Geometry: final body of the model. Coordinates: model frame, mm. A direction names the side the tool comes from. Round coordinates to 2 decimals unless told otherwise and drop trailing zeros. Write each loop counter-clockwise with the first axis right and the second up, starting at its lowest first coordinate (ties: lowest second). Pieces come first, ordered by that corner, then holes. Notation, with made-up numbers: (-9.5, -27) - (49.5, -27) arc R22 cw to (49.5, -14) - close; hole circle Ø1 at (49, -20). An arc over 180 degrees is marked (long way). Use a Markdown table: item, result. Add a question column.
```python
from build123d import *

# Parameters (mm, degrees)
PAD_DEPTH     = 101.6
SKETCH001_W   = 2.54
SKETCH001_H   = 83.8962
SKETCH001_W_2 = 12.7
SKETCH001_H_2 = 50.8
SKETCH001_W_3 = 146.9
SKETCH001_H_3 = 2.54
PAD001_DEPTH  = 2.54
CHAMFER_SIZE  = 50.8
FILLET_R      = 1.27


with BuildPart() as part:
    # Sketch → Pad (new body)
    with BuildSketch(Plane.XY):
        Polygon((-2.54, 2.54), (-2.54, -121.9962), (0, -121.9962), (0, 0), (185, 0), (185, -121.9962), (187.54, -121.9962), (187.54, 2.54), align=None)
    extrude(amount=PAD_DEPTH)

    # Sketch001 → Pad001 (join)
    with BuildSketch(Plane.XY):
        with Locations((1.27, -60.9981)):
            Rectangle(SKETCH001_W, SKETCH001_H)
        with Locations((178.65, -76.2)):
            Rectangle(SKETCH001_W_2, SKETCH001_H_2)
        with Locations((92.5, -1.27)):
            Rectangle(SKETCH001_W_3, SKETCH001_H_3)
    extrude(amount=PAD001_DEPTH)

    # Chamfer
    chamfer_edges = [part.edges().sort_by_distance(p)[0] for p in [
        (-1.27, -121.9962, 101.6),
        (186.27, -121.9962, 101.6),
    ]]
    chamfer(chamfer_edges, length=CHAMFER_SIZE)

    # Fillet
    fillet_edges = [part.edges().sort_by_distance(p)[0] for p in [
        (185, 0, 50.8),
        (0, 0, 50.8),
        (-2.54, 2.54, 50.8),
        (187.54, 2.54, 50.8),
    ]]
    fillet(fillet_edges, radius=FILLET_R)


solid = part.part
```
1) Pin query (flat end, axial travel): P1, Ø6, axis at x = 22, z = 36.5, coming from the -Y side; P2, Ø0.8, axis at x = 126.5, y = -1.5, coming from the +Z side; P3, Ø2, axis at x = 105, z = 1, coming from the -Y side. Return the tip coordinate at first contact, or that it passes through.
2) Section C-C, the plane z = 31.5. Return the cut outline in (x, y), then the cut area to 3 significant figures.
3) Set-up query: faces 1 (the flat face through (179, -76, 2.54)), 2 (the flat face through (186.252, -96.952, 75.844)). Return all of +Z, -Z, +X, -X, +Y, -Y with unobstructed straight access to the full face (end or side cutting, diameter ignored); none if empty.
4) Section B-B, the plane y = -62.5. Return the cut outline in (x, z).
5) Draft query along X for faces 3 (the flat face through (94, 2.54, 50)), 4 (the flat face through (187.54, -61, 50)), 5 (the flat face through (0, -62, 50)). Return one class per face: released by +X, released by -X, zero draft, split by the parting line, or undercut.
6) Section D-D, the plane x = 122.5. Return the cut outline in (y, z).
7) Section A-A, the plane y = -14.5. Return the cut outline in (x, z), then the cut area to 3 significant figures.
8) Material intervals for L1, parallel to X at y = -110.5, z = 45.5; L2, parallel to Y at x = 147, z = 46.5, sorted ascending. Write a range as from..to.
Output values:
| question | item | result |
|---|---|---|
| 1 | P1 | stops at y = 0 |
| 1 | P2 | stops at z = 2.54 |
| 1 | P3 | stops at y = -2.54 |
| 2 | outline | (-2.54, -122) - (0, -122) - (0, -1.27) arc R1.27 cw to (1.27, 0) - (183.73, 0) arc R1.27 cw to (185, -1.27) - (185, -122) - (187.54, -122) - (187.54, 1.27) arc R1.27 ccw to (186.27, 2.54) - (-1.27, 2.54) arc R1.27 ccw to (-2.54, 1.27) - close |
| 2 | area | 1,100 mm^2 |
| 3 | face 1 | +Z, -Y |
| 3 | face 2 | +Z, +X, -X, -Y |
| 4 | outline | (-2.54, 0) - (2.54, 0) - (2.54, 2.54) - (0, 2.54) - (0, 101.6) - (-2.54, 101.6) - close; (172.3, 0) - (187.54, 0) - (187.54, 101.6) - (185, 101.6) - (185, 2.54) - (172.3, 2.54) - close |
| 5 | face 3 | zero draft |
| 5 | face 4 | released by +X |
| 5 | face 5 | undercut |
| 6 | outline | (-2.54, 0) - (2.54, 0) - (2.54, 101.6) - (0, 101.6) - (0, 2.54) - (-2.54, 2.54) - close |
| 7 | outline | (-2.54, 0) - (0, 0) - (0, 101.6) - (-2.54, 101.6) - close; (185, 0) - (187.54, 0) - (187.54, 101.6) - (185, 101.6) - close |
| 7 | area | 516 mm^2 |
| 8 | L1 | x = -2.54..0, 185..187.54 |
| 8 | L2 | y = 0..2.54 |
